The model under review builds one solid part; all positions refer to its coordinate system, in mm. A direction names the side the tool comes from. Coordinates: 2 decimals unless noted, no trailing zeros. Loops run counter-clockwise (first coordinate to the right, second up) from the corner with the lowest first, then second, coordinate; pieces in that order, holes last. Notation, with made-up numbers: M 0.25,1.5 L 55.25,1.5 A17 ccw 55.25,15.5 Z; hole C -21.5,13.25 d4. An arc over 180 degrees is marked long. Return JSON: item names as keys, results as strings.
```python
from build123d import *

# Parameters (mm, degrees)
F1_DEPTH = 34.925
F0_W     = 12.7
F0_H     = 44.45
F0_R     = 1.5875
F2_DEPTH = 1.5875
F3_W     = 41.275
F3_H     = 15.875
F4_DEPTH = 11.1125
F5_R     = 5.55625
F6_DEPTH = 3.175


# Not quite as in the source:
# - a fillet or chamfer that OpenCascade refuses, or shapes differently, is made with other operations: its cross-section is extruded or revolved along the edge and cut away or added


with BuildPart() as f1:
    # F0 (on Top) → F1 (new body)
    with BuildSketch(Plane.XY):
        Polygon((34.13125, 22.225), (34.13125, 52.3875), (-34.13125, 52.3875), (-34.13125, 22.225), (-34.13125, -22.225), (-34.13125, -52.3875), (34.13125, -52.3875), (34.13125, -22.225), align=None)
    extrude(amount=F1_DEPTH)

    # F0 (on Top) → F2 (join)
    with BuildSketch(Plane.XY):
        with Locations((-40.48125, 0)):
            Rectangle(F0_W, F0_H)
        with Locations((-40.48125, -15.875)):
            Circle(F0_R, mode=Mode.SUBTRACT)
        with BuildLine():
            Line((-38.89375, 0.425369343), (-38.89375, -2.749630657))
            ThreePointArc((-38.89375, -2.749630657), (-40.48125, -4.337130657), (-42.06875, -2.749630657))
            Line((-42.06875, -2.749630657), (-42.06875, 0.425369343))
            ThreePointArc((-42.06875, 0.425369343), (-40.48125, 6.35), (-38.89375, 0.425369343))
        make_face(mode=Mode.SUBTRACT)
        with Locations((-40.48125, 15.875)):
            Circle(F0_R, mode=Mode.SUBTRACT)
        with Locations((40.48125, 0)):
            Rectangle(F0_W, F0_H)
        with Locations((40.48125, -15.875)):
            Circle(F0_R, mode=Mode.SUBTRACT)
        with BuildLine():
            ThreePointArc((38.89375, 0.425369343), (40.48125, 6.35), (42.06875, 0.425369343))
            Line((42.06875, 0.425369343), (42.06875, -2.749630657))
            ThreePointArc((42.06875, -2.749630657), (40.48125, -4.337130657), (38.89375, -2.749630657))
            Line((38.89375, -2.749630657), (38.89375, 0.425369343))
        make_face(mode=Mode.SUBTRACT)
        with Locations((40.48125, 15.875)):
            Circle(F0_R, mode=Mode.SUBTRACT)
    extrude(amount=F2_DEPTH)

    # F3 (on face) → F4 (join)
    with BuildSketch(Plane(origin=(0, 52.3875, 0), x_dir=(-1, 0, 0), z_dir=(0, 1, 0))):
        with Locations((0, 17.4625)):
            Rectangle(F3_W, F3_H)
    extrude(amount=F4_DEPTH)

    # F5 (on face) → F6 (join)
    with BuildSketch(Plane.XZ.offset(52.3875)):
        with Locations((19.84375, 19.05)):
            Circle(F5_R)
    extrude(amount=F6_DEPTH)

    # F7: fillet of radius 5.08 on 1 edges, made by hand

    # F7_s1 → F7_t2 (revolve, cut)
    with BuildSketch(Plane.XY.offset(19.05)):
        with BuildLine():
            ThreePointArc((25.4, -52.3875), (23.5305202921, -54.6946134838), (20.6907139607, -55.5625))
            Line((20.6907139607, -55.5625), (25.4, -55.5625))
            Line((25.4, -55.5625), (25.4, -52.3875))
        make_face()
    revolve(axis=Axis((19.84375, -55.5625, 19.05), (0, -1, 0)), mode=Mode.SUBTRACT)


solid = f1.part
```
1. Add section B-B on y = -9. Give the boundary of the cut face in (x, z) (1 decimal).
Check values:
{"outline": "M -46.8,0 L 46.8,0 L 46.8,1.6 L 34.1,1.6 L 34.1,34.9 L -34.1,34.9 L -34.1,1.6 L -46.8,1.6 Z"}
2. Add section D-D on z = 27. Give the boundary of the cut face in (x, y).
Check values:
{"outline": "M -34.13,-52.39 L 34.13,-52.39 L 34.13,52.39 L -34.13,52.39 Z"}
3. Machinability: for faces 5 (the face through (0, 58, 25.4)), 6 (the face through (20.638, 58, 17)), 7 (the face through (38, 0, 1.588)), 8 (the face through (0, 58, 9.525)), 9 (the face through (-20.638, 58, 17)), which of the approach directions +Z, -Z, +X, -X, +Y, -Y give a long, thin tool a straight path to every point of the face, cutting with its end or side? Answer none if there is none.
Check values:
{"face 5": "+Z, +X, -X, +Y", "face 6": "+Z, -Z, +X, +Y", "face 7": "+Z, +X, +Y, -Y", "face 8": "-Z, +X, -X, +Y", "face 9": "+Z, -Z, -X, +Y"}
4. Add section A-A on x = -40.5. Give the boundary of the cut face in (y, z) (1 decimal).
Check values:
{"outline": "M -22.2,0 L -17.5,0 L -17.5,1.6 L -22.2,1.6 Z; M -14.3,0 L -4.3,0 L -4.3,1.6 L -14.3,1.6 Z; M 6.3,0 L 14.3,0 L 14.3,1.6 L 6.3,1.6 Z; M 17.5,0 L 22.2,0 L 22.2,1.6 L 17.5,1.6 Z"}
5. Add section C-C on x = -1.5. Give the boundary of the cut face in (y, z) (1 decimal), plus the area to 3 significant figures.
Check values:
{"outline": "M -52.4,0 L 52.4,0 L 52.4,9.5 L 63.5,9.5 L 63.5,25.4 L 52.4,25.4 L 52.4,34.9 L -52.4,34.9 Z", "area": "3,840 mm²"}
6. Insertion check: pin 1 Ø8 at (y, z) = (-29, 19) entering from -X; pin 2 Ø12 at (y, z) = (58.5, 16) entering from +X; pin 3 Ø1 at (y, z) = (-27, 25.5) entering from +X. Each pin has a flat end and moves straight along its axis. Give the tip position at first contact, or say it passes through.
Check values:
{"pin 1": "x = -34.13", "pin 2": "x = 20.64", "pin 3": "x = 34.13"}
7. To check wall thickness, follow line 1 (X direction, y = 17.5, z = 32); line 2 (Y direction, x = -9.5, z = 24); line 3 (Y direction, x = -0.5, z = 29). State the ranges of each line that lie inside material, in increasing order.
Check values:
{"line 1": "-34.13 to 34.13", "line 2": "-52.39 to 63.5", "line 3": "-52.39 to 52.39"}
8. The part is to be moulded in two halves that separate along X. For faces 1 (the face through (40.365, 6.348, 0.783)), 2 (the face through (-43, 0, 1.588)), 3 (the face through (-41.74, 14.91, 0.78)), 4 (the face through (34.131, -1, 17)), say which applies: released by +X, released by -X, zero draft, split by the parting line, or undercut.
Check values:
{"face 1": "undercut", "face 2": "zero draft", "face 3": "undercut", "face 4": "released by +X"}
